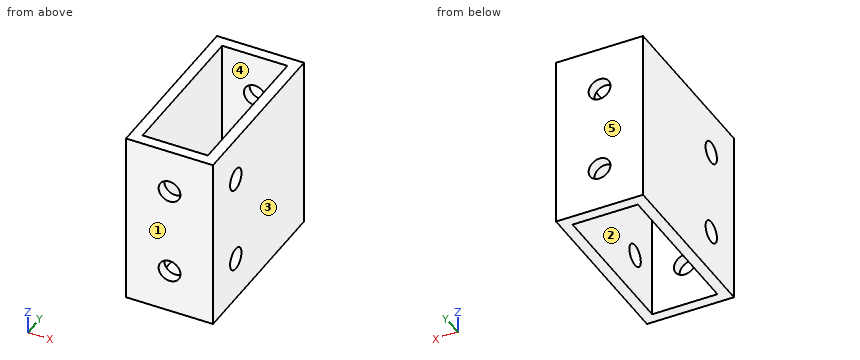
from build123d import *

# Parameters (mm, degrees)
SKETCH1_W           = 25.4
SKETCH1_H           = 50.8
SKETCH1_W_2         = 19.05
SKETCH1_H_2         = 44.45
BOSS_EXTRUDE1_DEPTH = 50.8
SKETCH2_R           = 3.175
CUT_EXTRUDE1_DEPTH  = 50.8
SKETCH3_R           = 3.175
CUT_EXTRUDE2_DEPTH  = 50.8


with BuildPart() as part:
    # Sketch1 → Boss-Extrude1 (new body)
    with BuildSketch(Plane.XY):
        with Locations((12.7, 25.4)):
            Rectangle(SKETCH1_W, SKETCH1_H)
        with Locations((12.7, 25.4)):
            Rectangle(SKETCH1_W_2, SKETCH1_H_2, mode=Mode.SUBTRACT)
    extrude(amount=BOSS_EXTRUDE1_DEPTH)

    # Sketch2 → Cut-Extrude1 (cut)
    with BuildSketch(Plane.XZ):
        with Locations(Location((12.7, 38.1, 0), (0, 0, 270))):
            Circle(SKETCH2_R)
        with Locations(Location((12.7, 12.7, 0), (0, 0, 270))):
            Circle(SKETCH2_R)
    extrude(amount=-CUT_EXTRUDE1_DEPTH, mode=Mode.SUBTRACT)

    # Sketch3 → Cut-Extrude2 (cut)
    with BuildSketch(Plane.ZY):
        with Locations((38.1, 12.7)):
            Circle(SKETCH3_R)
        with Locations((12.7, 12.7)):
            Circle(SKETCH3_R)
    extrude(amount=-CUT_EXTRUDE2_DEPTH, mode=Mode.SUBTRACT)


solid = part.part
For this review, take the finished solid that the model builds, in its own axes (mm). Face numbers are marked on the shaded views. A direction names the side the tool comes from. Round coordinates to 2 decimals unless told otherwise and drop trailing zeros. Write each loop counter-clockwise with the first axis right and the second up, starting at its lowest first coordinate (ties: lowest second). Pieces come first, ordered by that corner, then holes. Notation, with made-up numbers: (-14, -36) -> (-9, -36) arc R5 cw to (-9, -27) -> close; hole circle Ø1 at (-32.75, 24). An arc over 180 degrees is marked (long way). Put each result on its own line as item: value.
Q1. Consider section C-C on y = 22.5. State the section outline as (x, z) points (3 decimals).
Determined:
outline: (0, 0) -> (3.175, 0) -> (3.175, 50.8) -> (0, 50.8) -> close; (22.225, 0) -> (25.4, 0) -> (25.4, 50.8) -> (22.225, 50.8) -> close
Q2. Machinability: for the marked faces 1 and 2, which of the approach directions +Z, -Z, +X, -X, +Y, -Y give a long, thin tool a straight path to every point of the face, cutting with its end or side? Answer none if there is none.
Determined:
face 1: +Z, -Z, +X, -X, -Y
face 2: +Z, -Z
Q3. Consider section B-B on z = 7.5. State the section outline as (x, y) points (3 decimals).
Determined:
outline: (0, 0) -> (25.4, 0) -> (25.4, 50.8) -> (0, 50.8) -> close; hole (3.175, 3.175) -> (22.225, 3.175) -> (22.225, 47.625) -> (3.175, 47.625) -> close
Q4. Consider section D-D on z = 38.1. State the section outline as (x, y) points (3 decimals).
Determined:
outline: (0, 0) -> (9.525, 0) -> (9.525, 3.175) -> (3.175, 3.175) -> (3.175, 9.525) -> (0, 9.525) -> close; (0, 15.875) -> (3.175, 15.875) -> (3.175, 47.625) -> (9.525, 47.625) -> (9.525, 50.8) -> (0, 50.8) -> close; (15.875, 0) -> (25.4, 0) -> (25.4, 9.525) -> (22.225, 9.525) -> (22.225, 3.175) -> (15.875, 3.175) -> close; (15.875, 47.625) -> (22.225, 47.625) -> (22.225, 15.875) -> (25.4, 15.875) -> (25.4, 50.8) -> (15.875, 50.8) -> close
Q5. Consider section A-A on y = 12.7. State the section outline as (x, z) points (3 decimals).
Determined:
outline: (0, 0) -> (3.175, 0) -> (3.175, 9.525) -> (0, 9.525) -> close; (0, 15.875) -> (3.175, 15.875) -> (3.175, 34.925) -> (0, 34.925) -> close; (0, 41.275) -> (3.175, 41.275) -> (3.175, 50.8) -> (0, 50.8) -> close; (22.225, 0) -> (25.4, 0) -> (25.4, 9.525) -> (22.225, 9.525) -> close; (22.225, 15.875) -> (25.4, 15.875) -> (25.4, 34.925) -> (22.225, 34.925) -> close; (22.225, 41.275) -> (25.4, 41.275) -> (25.4, 50.8) -> (22.225, 50.8) -> close
Q6. The part is to be moulded in two halves that separate along X. For the marked faces 3, 4 and 5, say which applies: released by +X, released by -X, zero draft, split by the parting line, or undercut.
Determined:
face 3: released by +X
face 4: undercut
face 5: zero draft
Q7. To check wall thickness, follow L1, parallel to Y at x = 11.25, z = 8 (3 decimals); L2, parallel to X at y = 37.5, z = 19.5 (3 decimals); L3, parallel to Y at x = 1.35, z = 38.1 (3 decimals). State the ranges of each line that lie inside material, in increasing order. Write a range as [from, to].
Determined:
L1: y = [0, 3.175], [47.625, 50.8]
L2: x = [0, 3.175], [22.225, 25.4]
L3: y = [0, 9.525], [15.875, 50.8]
